Part print with two shaded views. Sizes in mm from the minimum x, y, z corner. Round coordinates to 2 decimals unless told otherwise and drop trailing zeros. Order: outer loops, then holes, each group sorted by start corner. A loop starts at its lowest first (then second) coordinate and runs counter-clockwise, first axis right, second up. Notation, with made-up numbers: M 18,84.25 L 36,84.25 A17 cw 36,101.25 Z; hole C -17.5,-38 d3. An arc over 180 degrees is marked long. Return JSON: item names as keys, results as strings. Group by question number.
Item 1: Slice it at A-A on y = 10.5. Write the cut outline in (x, z), then the cut area to 3 significant figures.
Item 2: Probe line 1 along X through (y, z) = (33.5, 4.75); line 2 along Z through (x, y) = (34.5, 29.5); line 3 along Z through (x, y) = (62, 41.5). List the from-to ranges inside material, lowest first.
Item 3: Slice it at D-D on y = 45. Write the cut outline in (x, z), then the cut area to 3 significant figures.
Item 4: Slice it at B-B on x = 18. Write the cut outline in (y, z).
Item 5: Pull direction X, two halves, no side cores. Call the marked faces 1, 2, 3 and 4: pulls with the +X half, pulls with the -X half, needs draft (parallel to the pull), parting line crosses it, or undercut.
Item 6: Pin check, flat tips, straight feed: pin 1 Ø10 at (x, z) = (67.5, 10.5) entering from -Y; pin 2 Ø6 at (x, z) = (131.5, 13.5) entering from +Y. Stop position of each tip, or through.
Item 7: Slice it at C-C on z = 14.5. Write the cut outline in (x, y).
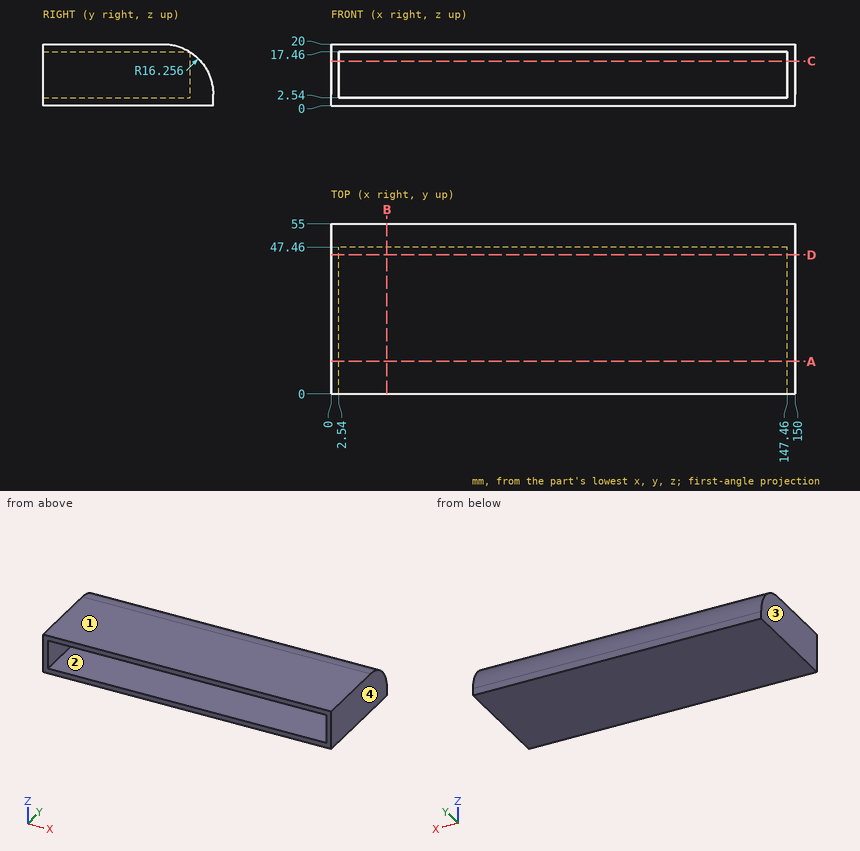
Output values:
{
 "1": {"outline": "M 0,0 L 150,0 L 150,20 L 0,20 Z; hole M 2.54,2.54 L 147.46,2.54 L 147.46,17.46 L 2.54,17.46 Z", "area": "838 mm²"},
 "2": {"line 1": "0 to 2.54, 147.46 to 150", "line 2": "0 to 2.54, 17.46 to 20", "line 3": "0 to 2.54, 17.46 to 19.76"},
 "3": {"outline": "M 0,0 L 150,0 L 150,18.75 L 0,18.75 Z; hole M 2.54,2.54 L 147.46,2.54 L 147.46,17.46 L 2.54,17.46 Z", "area": "650 mm²"},
 "4": {"outline": "M 0,0 L 55,0 L 55,3.74 A16.26 ccw 38.74,20 L 0,20 L 0,17.46 L 47.46,17.46 L 47.46,2.54 L 0,2.54 Z"},
 "5": {"face 1": "needs draft", "face 2": "undercut", "face 3": "pulls with the -X half", "face 4": "pulls with the +X half"},
 "6": {"pin 1": "y = 47.46", "pin 2": "y = 53.53"},
 "7": {"outline": "M 0,0 L 2.54,0 L 2.54,47.46 L 147.46,47.46 L 147.46,0 L 150,0 L 150,50.93 L 0,50.93 Z"}
}
